from build123d import *

# Parameters (mm, degrees)
SKETCH1_W                    = 43
SKETCH1_H                    = 58
BOSS_EXTRUDE1_DEPTH          = 2
CUT_EXTRUDE1_DEPTH           = 3
CUT_EXTRUDE2_DEPTH           = 3
SKETCH4_W                    = 1
SKETCH4_H                    = 31
BOSS_EXTRUDE2_DEPTH          = 5
SKETCH5_W                    = 1
SKETCH5_H                    = 31
BOSS_EXTRUDE3_DEPTH          = 5
DRAFT1_ANGLE                 = 15
F_8_0_8_DIAMETER_HOLE1_D     = 8
F_8_0_8_DIAMETER_HOLE1_DEPTH = 7


with BuildPart() as part:
    # Sketch1 → Boss-Extrude1 (new body)
    with BuildSketch(Plane(origin=(0, 0, -2), x_dir=(-1, 0, 0), z_dir=(0, 0, -1))):
        Rectangle(SKETCH1_W, SKETCH1_H)
    extrude(amount=-BOSS_EXTRUDE1_DEPTH)

    # Sketch2 → Cut-Extrude1 (cut, through all)
    with BuildSketch(Plane.XY):
        with BuildLine():
            Line((4.25, 29), (-4.25, 29))
            Line((-4.25, 29), (-4.25, 23.75))
            ThreePointArc((-4.25, 23.75), (0, 19.5), (4.25, 23.75))
            Line((4.25, 23.75), (4.25, 29))
        make_face()
    extrude(amount=-CUT_EXTRUDE1_DEPTH, mode=Mode.SUBTRACT)

    # Sketch3 → Cut-Extrude2 (cut, through all)
    with BuildSketch(Plane.XY):
        with BuildLine():
            Line((-4.25, -29), (4.25, -29))
            Line((4.25, -29), (4.25, -23.75))
            ThreePointArc((4.25, -23.75), (0, -19.5), (-4.25, -23.75))
            Line((-4.25, -23.75), (-4.25, -29))
        make_face()
    extrude(amount=-CUT_EXTRUDE2_DEPTH, mode=Mode.SUBTRACT)

    # Sketch4 → Boss-Extrude2 (add)
    with BuildSketch(Plane(origin=(0, 0, -2), x_dir=(-1, 0, 0), z_dir=(0, 0, -1))):
        with Locations((-21, 0)):
            Rectangle(SKETCH4_W, SKETCH4_H)
    extrude(amount=BOSS_EXTRUDE2_DEPTH)

    # Sketch5 → Boss-Extrude3 (add)
    with BuildSketch(Plane(origin=(0, 0, -2), x_dir=(-1, 0, 0), z_dir=(0, 0, -1))):
        with Locations((21, 0)):
            Rectangle(SKETCH5_W, SKETCH5_H)
    extrude(amount=BOSS_EXTRUDE3_DEPTH)

    # Draft1
    draft1_faces = [part.faces().sort_by_distance(p)[0] for p in [
        (21, -15.5, -4.5),
        (21, 15.5, -4.5),
        (-21, 15.5, -4.5),
        (-21, -15.5, -4.5),
    ]]
    draft(draft1_faces, Plane(origin=(0, 0, -2), x_dir=(-1, 0, 0), z_dir=(0, 0, -1)), DRAFT1_ANGLE)

    # Ø8.0 (8) Diameter Hole1
    with Locations(Plane.XY):
        with Locations((12.5, 22), (-12.5, 22), (-12.5, -22), (12.5, -22)):
            Hole(F_8_0_8_DIAMETER_HOLE1_D / 2, depth=F_8_0_8_DIAMETER_HOLE1_DEPTH)


solid = part.part
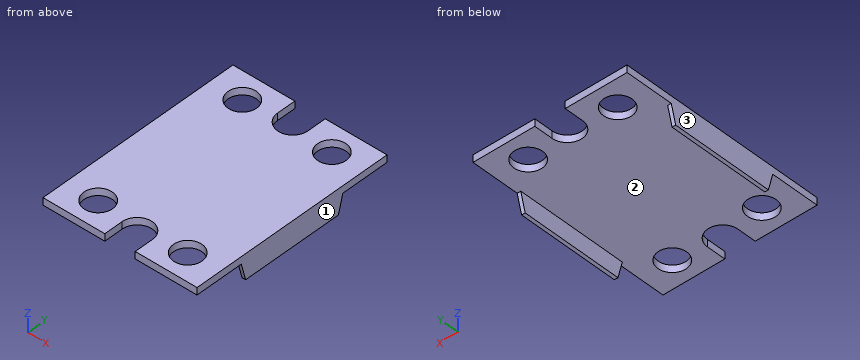
The listing builds one solid part. Answer for the finished solid, in the listing's coordinates (mm). Face numbers are marked on the shaded views. Give positions to 0.01 mm unless a question says otherwise; leave off trailing zeros. Write each loop counter-clockwise with the first axis right and the second up, starting at its lowest first coordinate (ties: lowest second). Pieces come first, ordered by that corner, then holes.
1) Section D-D (y = 2) is taken. Write down the section's boundary in (x, z).
2) Find the intervals of material crossed by L1, parallel to Y at x = 12.5, z = -1.45; L2, parallel to X at y = 4, z = -4; L3, parallel to Z at x = -10.5, y = 4, in increasing order.
3) Section A-A (x = -12.5) is taken. Write down the section's boundary in (y, z).
4) Given P1, Ø1, axis at x = -7, y = 0, coming from the -Z side; P2, Ø3, axis at x = 16.5, y = 13.5, coming from the +Z side; P3, Ø6.5, axis at x = -12.5, y = -22, coming from the -Z side, each flat-ended and moving along its own axis, determine where each tip first touches the part or whether it passes through.
5) Section C-C (y = -22) is taken. Write down the section's boundary in (x, z), and give its area (3 significant figures).
6) Section B-B (z = -1) is taken. Write down the section's boundary in (x, y).
7) For a pull along X with two mould halves and no side action, classify the marked faces 1, 2 and 3 as pulls with the +X half, pulls with the -X half, needs draft (parallel to the pull), parting line crosses it, or undercut.
Response:
1. outline: (-21.5, -7) - (-20.5, -7) - (-20.5, -2) - (20.5, -2) - (20.5, -7) - (21.5, -7) - (21.5, 0) - (-21.5, 0) - close
2. L1: y = -29 to -26, -18 to 18, 26 to 29
2. L2: x = -21.5 to -20.5, 20.5 to 21.5
2. L3: z = -2 to 0
3. outline: (-29, -2) - (-26, -2) - (-26, 0) - (-29, 0) - close; (-18, -2) - (18, -2) - (18, 0) - (-18, 0) - close; (26, -2) - (29, -2) - (29, 0) - (26, 0) - close
4. P1: stops at z = -2
4. P2: stops at z = 0
4. P3: passes through
5. outline: (-21.5, -2) - (-16.5, -2) - (-16.5, 0) - (-21.5, 0) - close; (-8.5, -2) - (-3.87, -2) - (-3.87, 0) - (-8.5, 0) - close; (3.87, -2) - (8.5, -2) - (8.5, 0) - (3.87, 0) - close; (16.5, -2) - (21.5, -2) - (21.5, 0) - (16.5, 0) - close
5. area: 38.5 mm2
6. outline: (-21.5, -29) - (-4.25, -29) - (-4.25, -23.75) arc R4.25 cw to (4.25, -23.75) - (4.25, -29) - (21.5, -29) - (21.5, 29) - (4.25, 29) - (4.25, 23.75) arc R4.25 cw to (-4.25, 23.75) - (-4.25, 29) - (-21.5, 29) - close; hole circle Ø8 at (-12.5, -22); hole circle Ø8 at (-12.5, 22); hole circle Ø8 at (12.5, -22); hole circle Ø8 at (12.5, 22)
7. face 1: pulls with the +X half
7. face 2: undercut
7. face 3: pulls with the -X half
